Geometry: see drawing. Coordinates: mm, zero at the bounding-box minimum. Coordinates: 2 decimals unless noted, no trailing zeros. Loops run counter-clockwise (first coordinate to the right, second up) from the corner with the lowest first, then second, coordinate; pieces in that order, holes last. Notation, with made-up numbers: (-32, 17) -> (-21, 17) arc R20 ccw to (-21, 39) -> close; hole circle Ø5 at (65.25, -28). An arc over 180 degrees is marked (long way). Answer as a JSON object with one key per item and string values.
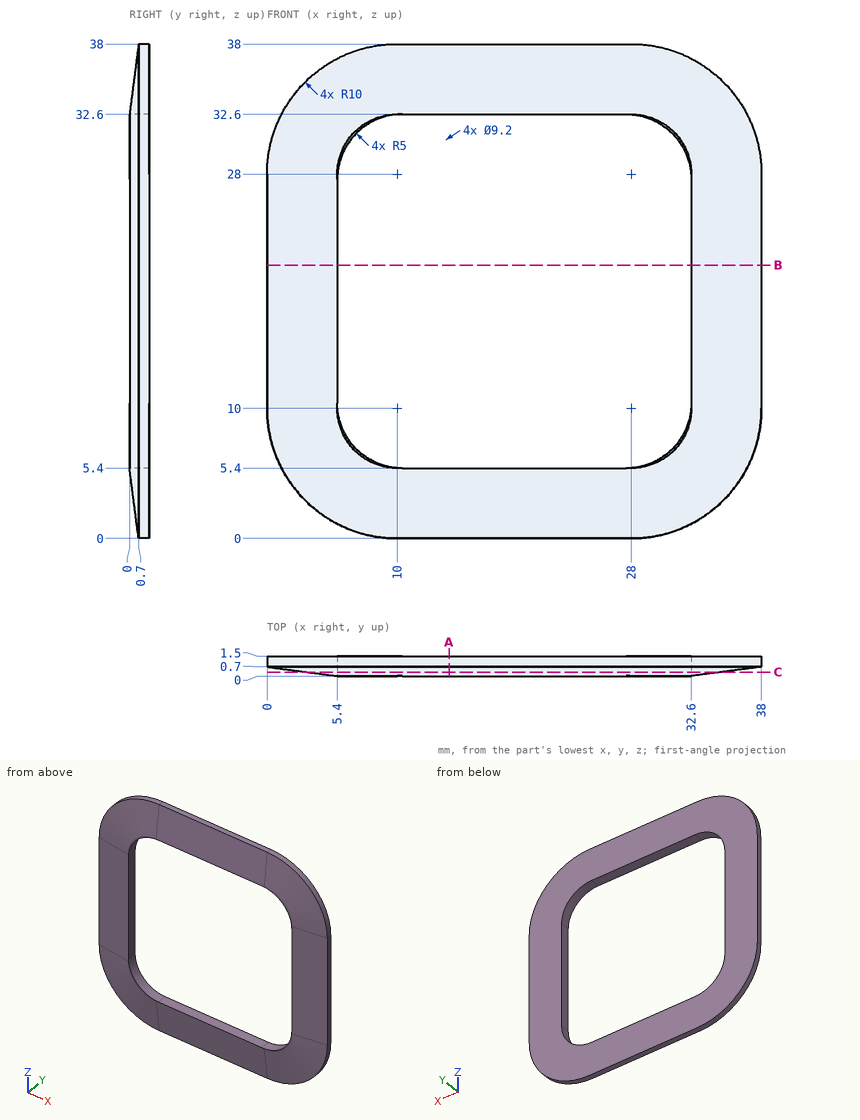
1. Pin query (flat end, axial travel): P1, Ø4, axis at x = 7, z = 4.5, coming from the -Y side; P2, Ø1.5, axis at x = 6, z = 33.5, coming from the -Y side. Return the tip coordinate at first contact, or that it passes through.
Reply:
{"P1": "stops at y = 0", "P2": "stops at y = 0.19"}
2. Section query A-A (x = 14). Return loops of the section in (y, z), plus the area to 3 significant figures.
Reply:
{"outline": "(0, 5.4) -> (0.7, 0) -> (1.5, 0) -> (1.5, 5.4) -> close; (0, 32.6) -> (1.5, 32.6) -> (1.5, 38) -> (0.7, 38) -> close", "area": "12.4 mm2"}
3. Line query: line 1 along X through (y, z) = (0.9, 17); line 2 along Z through (x, y) = (7.5, 1.15). Output: solid intervals per line, ascending.
Reply:
{"line 1": "x = 0 to 5.4, 32.6 to 38", "line 2": "z = 0.32 to 6.33, 31.67 to 37.68"}
4. Section query C-C (y = 0.3). Return loops of the section in (x, z).
Reply:
{"outline": "(3.09, 10) arc R6.91 ccw to (10, 3.09) -> (28, 3.09) arc R6.91 ccw to (34.91, 10) -> (34.91, 28) arc R6.91 ccw to (28, 34.91) -> (10, 34.91) arc R6.91 ccw to (3.09, 28) -> close; hole (5.4, 10.4) arc R5 ccw to (10.4, 5.4) -> (27.6, 5.4) arc R5 ccw to (32.6, 10.4) -> (32.6, 27.6) arc R5 ccw to (27.6, 32.6) -> (10.4, 32.6) arc R5 ccw to (5.4, 27.6) -> close"}
5. Section query B-B (z = 21). Return loops of the section in (x, y).
Reply:
{"outline": "(0, 0.7) -> (5.4, 0) -> (5.4, 1.5) -> (0, 1.5) -> close; (32.6, 0) -> (38, 0.7) -> (38, 1.5) -> (32.6, 1.5) -> close"}
